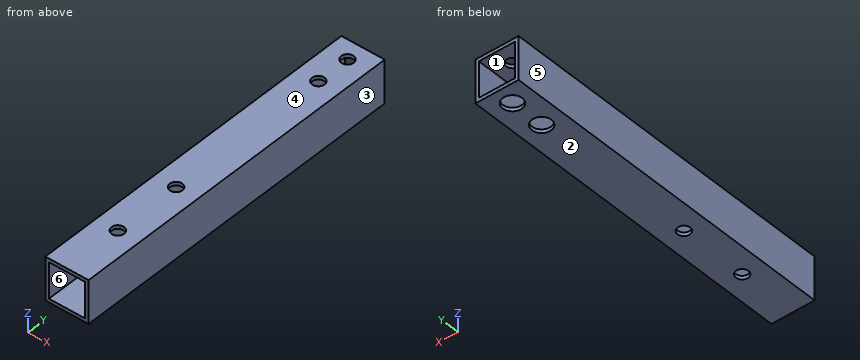
from build123d import *

# Parameters (mm, degrees)
SKETCH1_W           = 19.05
SKETCH1_H           = 19.05
SKETCH1_W_2         = 15.875
SKETCH1_H_2         = 15.875
BOSS_EXTRUDE1_DEPTH = 914.4
SKETCH2_R           = 2.75
CUT_EXTRUDE1_DEPTH  = 20.05
CUT_EXTRUDE2_REACH  = 21.05
SKETCH3_R           = 4.255
SKETCH4_W           = 19.05
SKETCH4_H           = 762
CUT_EXTRUDE3_DEPTH  = 20.05
SKETCH5_R           = 2.75
CUT_EXTRUDE4_DEPTH  = 20.05


with BuildPart() as part:
    # Sketch1 → Boss-Extrude1 (new body)
    with BuildSketch(Plane(origin=(0, 0, 0), x_dir=(1, 0, 0), z_dir=(0, 1, 0))):
        with Locations((9.525, 9.525)):
            Rectangle(SKETCH1_W, SKETCH1_H)
        with Locations((9.525, 9.525)):
            Rectangle(SKETCH1_W_2, SKETCH1_H_2, mode=Mode.SUBTRACT)
    extrude(amount=BOSS_EXTRUDE1_DEPTH)

    # Sketch2 → Cut-Extrude1 (cut, through all)
    with BuildSketch(Plane.XY):
        with Locations((9.525, 906.4)):
            Circle(SKETCH2_R)
        with Locations((9.525, 891.4)):
            Circle(SKETCH2_R)
    extrude(amount=-CUT_EXTRUDE1_DEPTH, mode=Mode.SUBTRACT)

    # Sketch3 → Cut-Extrude2 (cut, up to next)
    with BuildSketch(Plane(origin=(0, 0, -19.05), x_dir=(-1, 0, 0), z_dir=(0, 0, -1)), mode=Mode.PRIVATE) as cut_extrude2_sk1:
        with Locations((-9.525, 906.4)):
            Circle(SKETCH3_R)
    cut_extrude2_tool1 = extrude(cut_extrude2_sk1.sketch, amount=-CUT_EXTRUDE2_REACH, mode=Mode.PRIVATE) & part.part
    add(cut_extrude2_tool1.solids().sort_by_distance((9.525, 906.4, -19.05))[0], mode=Mode.SUBTRACT)
    # Sketch3 → Cut-Extrude2 (cut, up to next)
    with BuildSketch(Plane(origin=(0, 0, -19.05), x_dir=(-1, 0, 0), z_dir=(0, 0, -1)), mode=Mode.PRIVATE) as cut_extrude2_sk2:
        with Locations((-9.525, 891.4)):
            Circle(SKETCH3_R)
    cut_extrude2_tool2 = extrude(cut_extrude2_sk2.sketch, amount=-CUT_EXTRUDE2_REACH, mode=Mode.PRIVATE) & part.part
    add(cut_extrude2_tool2.solids().sort_by_distance((9.525, 891.4, -19.05))[0], mode=Mode.SUBTRACT)

    # Sketch4 → Cut-Extrude3 (cut, through all)
    with BuildSketch(Plane.XY):
        with Locations((9.525, 381)):
            Rectangle(SKETCH4_W, SKETCH4_H)
    extrude(amount=-CUT_EXTRUDE3_DEPTH, mode=Mode.SUBTRACT)

    # Sketch5 → Cut-Extrude4 (cut, through all)
    with BuildSketch(Plane.XY):
        with Locations((9.52, 788.2)):
            Circle(SKETCH5_R)
        with Locations((9.52, 818.2)):
            Circle(SKETCH5_R)
    extrude(amount=-CUT_EXTRUDE4_DEPTH, mode=Mode.SUBTRACT)


solid = part.part
The model under review builds one solid part; all positions refer to its coordinate system, in mm. Face numbers are marked on the shaded views. A direction names the side the tool comes from. Round coordinates to 2 decimals unless told otherwise and drop trailing zeros. Write each loop counter-clockwise with the first axis right and the second up, starting at its lowest first coordinate (ties: lowest second). Pieces come first, ordered by that corner, then holes. Notation, with made-up numbers: M -33.5,83.5 L 3.5,83.5 A19 ccw 3.5,119.5 Z; hole C 54.5,-7.75 d10. An arc over 180 degrees is marked long. Use a Markdown table: item, result. Add a question column.
Q1. We need section B-B, the plane z = -13. State the section outline as (x, y) points, plus the area to 3 significant figures.
Q2. We need section C-C, the plane y = 835.5. State the section outline as (x, z) points, plus the area to 3 significant figures.
Q3. The part is to be moulded in two halves that separate along Z. For the marked faces 1, 2, 3 and 4, say which applies: pulls with the +Z half, pulls with the -Z half, needs draft (parallel to the pull), parting line crosses it, or undercut.
Q4. Machinability: for the marked faces 5 and 6, which of the approach directions +Z, -Z, +X, -X, +Y, -Y give a long, thin tool a straight path to every point of the face, cutting with its end or side? Answer none if there is none.
Q5. We need section A-A, the plane y = 818.2. State the section outline as (x, z) points.
Q6. To check wall thickness, follow line 1 (Y direction, x = 9.52, z = -1.1); line 2 (Y direction, x = 9.52, z = -18.65) (3 decimals); line 3 (Z direction, x = 6.5, y = 873.5). State the ranges of each line that lie inside material, in increasing order.
Q7. Insertion check: pin 1 (7.5 mm diameter, centred on x = 9.525, y = 891.4, fed in from -Z); pin 2 (3.5 mm diameter, centred on x = 9.52, y = 788.2, fed in from -Z). Each pin has a flat end and moves straight along its axis. Give the tip position at first contact, or say it passes through.
Findings below:
| question | item | result |
|---|---|---|
| 1 | outline | M 0,762 L 1.59,762 L 1.59,914.4 L 0,914.4 Z; M 17.46,762 L 19.05,762 L 19.05,914.4 L 17.46,914.4 Z |
| 1 | area | 484 mm² |
| 2 | outline | M 0,-19.05 L 19.05,-19.05 L 19.05,0 L 0,0 Z; hole M 1.59,-17.46 L 17.46,-17.46 L 17.46,-1.59 L 1.59,-1.59 Z |
| 2 | area | 111 mm² |
| 3 | face 1 | undercut |
| 3 | face 2 | pulls with the -Z half |
| 3 | face 3 | needs draft |
| 3 | face 4 | pulls with the +Z half |
| 4 | face 5 | +Z, -Z, -X, +Y, -Y |
| 4 | face 6 | +Y, -Y |
| 5 | outline | M 0,-19.05 L 6.77,-19.05 L 6.77,-17.46 L 1.59,-17.46 L 1.59,-1.59 L 6.77,-1.59 L 6.77,0 L 0,0 Z; M 12.27,-19.05 L 19.05,-19.05 L 19.05,0 L 12.27,0 L 12.27,-1.59 L 17.46,-1.59 L 17.46,-17.46 L 12.27,-17.46 Z |
| 6 | line 1 | y = 762 to 785.45, 790.95 to 815.45, 820.95 to 888.65, 894.15 to 903.65, 909.15 to 914.4 |
| 6 | line 2 | y = 762 to 785.45, 790.95 to 815.45, 820.95 to 887.145, 895.655 to 902.145, 910.655 to 914.4 |
| 6 | line 3 | z = -19.05 to -17.46, -1.59 to 0 |
| 7 | pin 1 | stops at z = -1.59 |
| 7 | pin 2 | passes through |
